Can you work these out from the model? Positions are in its coordinate system, mm. Face numbers are marked on the shaded views. A direction names the side the tool comes from. Coordinates: 2 decimals unless noted, no trailing zeros. Order: outer loops, then holes, each group sorted by start corner. A loop starts at its lowest first (then second) coordinate and runs counter-clockwise, first axis right, second up. Notation, with made-up numbers: (34, -9) -> (87, -9) arc R13 ccw to (87, 6) -> close; hole circle Ø6 at (15.25, 28.5). An arc over 180 degrees is marked (long way). Write item = value, one per line. Start each with the question number.
from build123d import *

# Parameters (mm, degrees)
BOSS_EXTRUDE1_DEPTH = 15
SKETCH2_R           = 2.75
SKETCH2_R_2         = 3
SKETCH2_R_3         = 1.75
CUT_EXTRUDE1_DEPTH  = 15
SKETCH3_R           = 1.75
CUT_EXTRUDE2_DEPTH  = 23.5
CHAMFER1_SIZE       = 2


with BuildPart() as part:
    # Sketch1 → Boss-Extrude1 (new body)
    with BuildSketch(Plane.XY):
        Polygon((-2.135338346, 2.060150376), (1.864661654, 2.060150376), (1.864661654, -8.939849624), (20.364661654, -8.939849624), (20.364661654, -16.939849624), (-2.135338346, -16.939849624), align=None)
    extrude(amount=BOSS_EXTRUDE1_DEPTH)

    # Sketch2 → Cut-Extrude1 (cut)
    with BuildSketch(Plane.ZY.offset(2.135338346)):
        with Locations((7.5, -2.939849624)):
            Circle(SKETCH2_R)
        with Locations((11.5, -12.914706032)):
            Circle(SKETCH2_R_2)
        with Locations((11.5, -12.914706032)):
            Circle(SKETCH2_R_3, mode=Mode.SUBTRACT)
        with Locations((3.5, -12.914706032)):
            Circle(SKETCH2_R_2)
        with Locations((3.5, -12.914706032)):
            Circle(SKETCH2_R_3, mode=Mode.SUBTRACT)
    extrude(amount=-CUT_EXTRUDE1_DEPTH, mode=Mode.SUBTRACT)

    # Sketch3 → Cut-Extrude2 (cut, through all)
    with BuildSketch(Plane.ZY.offset(2.135338346)):
        with Locations((3.5, -12.914706032)):
            Circle(SKETCH3_R)
        with Locations((11.5, -12.914706032)):
            Circle(SKETCH3_R)
    extrude(amount=-CUT_EXTRUDE2_DEPTH, mode=Mode.SUBTRACT)

    # Chamfer1
    chamfer1_edges = [part.edges().sort_by_distance(p)[0] for p in [
        (-0.135338346, 2.060150376, 15),
        (-0.135338346, 2.060150376, 0),
    ]]
    chamfer(chamfer1_edges, length=CHAMFER1_SIZE)


solid = part.part
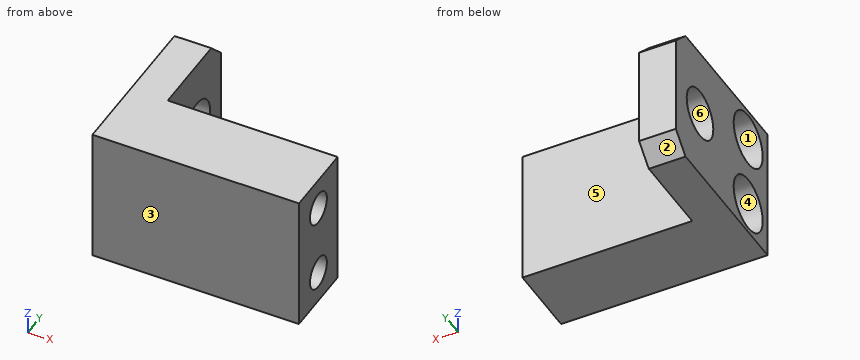
(1) For the marked faces 4, 5 and 6, which set-ups out of +Z, -Z, +X, -X, +Y, -Y let a thin tool reach every point of the face, with its end or its side?
(2) If I drill on L1, parallel to Y at x = 2, z = 3.5; L2, parallel to Y at x = 0.3, z = 7.5; L3, parallel to Z at x = 11.5, y = -13.5, over which ranges is the centre line in solid material (lowest first)? Write a range as from..to.
(3) Imagine slicing it at A-A (z = 11.5). Write out the boundary of the cut face in (x, y).
(4) For P1, Ø6, axis at x = 6, y = -2, coming from the -Z side; P2, Ø3, axis at y = -7.5, z = 9.5, coming from the +X side; P3, Ø3, axis at y = -12, z = 11, coming from the -X side; P4, Ø9, axis at y = -1.5, z = 10.5, coming from the +X side, each with a flat end and sliding along its axis, tell me the tip position at first contact or that it passes through.
(5) Imagine slicing it at C-C (z = 7.5). Write out the boundary of the cut face in (x, y).
(6) Thinking about a two-plate mould opening in Y: for the marked faces 1, 2 and 3, which applies, +Y half, -Y half, draft (parallel to the pull), parting line (faces both ways), or undercut?
(7) Imagine slicing it at B-B (x = 0.75). Write out the boundary of the cut face in (y, z).
(8) Imagine slicing it at D-D (x = 17.5). Write out the boundary of the cut face in (y, z).
Result set:
q1.face_4 = -X
q1.face_5 = +Z, -Z, +X, +Y
q1.face_6 = +X, -X
q2.L1 = -16.94..-15.91, -9.91..-8.94
q2.L2 = -16.94..-5.69, -0.19..2.06
q2.L3 = 0..0.56, 6.44..8.56, 14.44..15
q3.outline = (-2.14, -16.94) -> (20.36, -16.94) -> (20.36, -14.66) -> (12.86, -14.66) -> (12.86, -15.91) -> (-2.14, -15.91) -> close; (-2.14, -9.91) -> (12.86, -9.91) -> (12.86, -11.16) -> (20.36, -11.16) -> (20.36, -8.94) -> (1.86, -8.94) -> (1.86, 2.06) -> (-2.14, 2.06) -> close
q4.P1 = through
q4.P2 = 20.36
q4.P3 = 12.86
q4.P4 = 1.86
q5.outline = (-2.14, -16.94) -> (20.36, -16.94) -> (20.36, -8.94) -> (1.86, -8.94) -> (1.86, -5.69) -> (-2.14, -5.69) -> close; (-2.14, -0.19) -> (1.86, -0.19) -> (1.86, 2.06) -> (-2.14, 2.06) -> close
q6.face_1 = undercut
q6.face_2 = +Y half
q6.face_3 = -Y half
q7.outline = (-16.94, 0) -> (0.06, 0) -> (2.06, 2) -> (2.06, 13) -> (0.06, 15) -> (-16.94, 15) -> close; hole circle Ø6 at (-12.91, 3.5); hole circle Ø6 at (-12.91, 11.5); hole circle Ø5.5 at (-2.94, 7.5)
q8.outline = (-16.94, 0) -> (-8.94, 0) -> (-8.94, 15) -> (-16.94, 15) -> close; hole circle Ø3.5 at (-12.91, 3.5); hole circle Ø3.5 at (-12.91, 11.5)
